Source: three-view drawing plus pictorial views. Frame: mm from the lowest corner of the part. Round coordinates to 2 decimals unless told otherwise and drop trailing zeros. Write each loop counter-clockwise with the first axis right and the second up, starting at its lowest first coordinate (ties: lowest second). Pieces come first, ordered by that corner, then holes. Notation, with made-up numbers: M -7,-5 L 16,-5 A20 ccw 16,4 Z; hole C 1.25,-7 d5. An arc over 180 degrees is marked long. Answer as CSV lines item,"result". Start each with the question number.
Q1. Section query B-B on y = 38. Output: boundary loops of the cut face in (x, z).
Q2. Section query A-A on z = 63.2. Output: boundary loops of the cut face in (x, y).
Q3. First-contact query: pin 1 (12 mm diameter, centred on x = 375, z = 13.2, fed in from -Y). Flat tip, straight axial feed; report the tip coordinate or a pass-through.
Q4. Ray query, probe 1 along X at (y, z) = (11, 63); probe 2 along Z at (x, y) = (25, 18); probe 3 along X at (y, z) = (39, 67.5). Return the intervals inside material, ascending.
Q5. Section query C-C on x = 70. Output: boundary loops of the cut face in (y, z), and give its area (3 significant figures).
Q6. Section query D-D on z = 31. Output: boundary loops of the cut face in (x, y).
Q7. Mould query, pull axis Y, two halves, no side actions, for the marked faces 1, 2, 3 and 4. Classes: pulls with the +Y half, pulls with the -Y half, needs draft (parallel to the pull), parting line crosses it, or undercut.
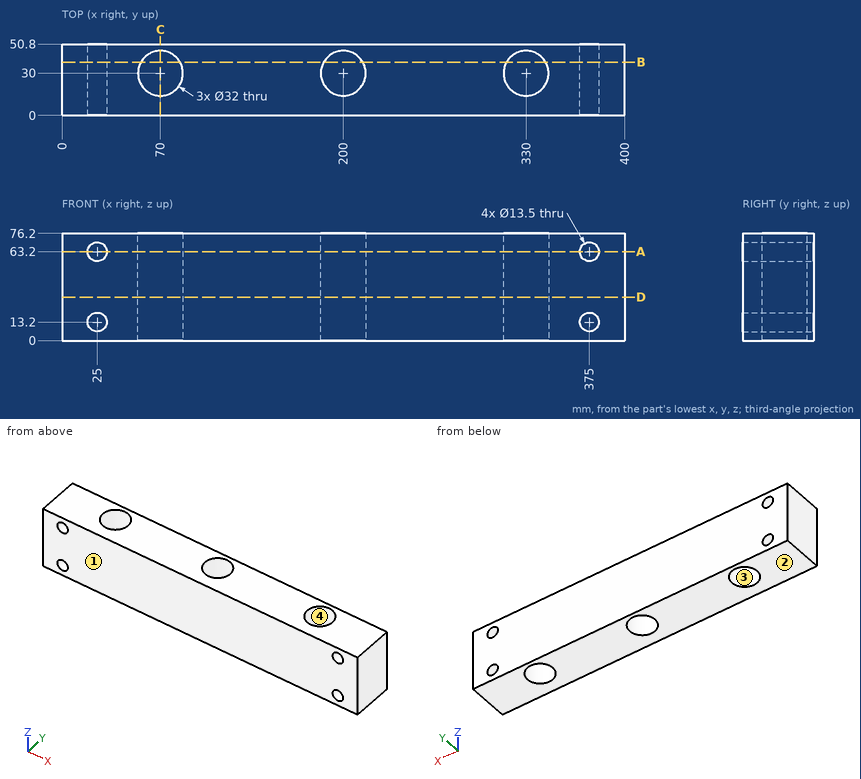
Entries:
1,outline,"M 0,0 L 56.14,0 L 56.14,76.2 L 0,76.2 Z; M 83.86,0 L 186.14,0 L 186.14,76.2 L 83.86,76.2 Z; M 213.86,0 L 316.14,0 L 316.14,76.2 L 213.86,76.2 Z; M 343.86,0 L 400,0 L 400,76.2 L 343.86,76.2 Z; hole C 25,13.2 d13.5; hole C 25,63.2 d13.5; hole C 375,13.2 d13.5; hole C 375,63.2 d13.5"
2,outline,"M 0,0 L 18.25,0 L 18.25,50.8 L 0,50.8 Z; M 31.75,0 L 368.25,0 L 368.25,50.8 L 31.75,50.8 Z; M 381.75,0 L 400,0 L 400,50.8 L 381.75,50.8 Z; hole C 70,30 d32; hole C 200,30 d32; hole C 330,30 d32"
3,pin 1,"passes through"
4,probe 1,"x = 0 to 18.25, 31.75 to 368.25, 381.75 to 400"
4,probe 2,"z = 0 to 6.45, 19.95 to 56.45, 69.95 to 76.2"
4,probe 3,"x = 0 to 19.8, 30.2 to 56.77, 83.23 to 186.77, 213.23 to 316.77, 343.23 to 369.8, 380.2 to 400"
5,outline,"M 0,0 L 14,0 L 14,76.2 L 0,76.2 Z; M 46,0 L 50.8,0 L 50.8,76.2 L 46,76.2 Z"
5,area,"1,430 mm^2"
6,outline,"M 0,0 L 400,0 L 400,50.8 L 0,50.8 Z; hole C 70,30 d32; hole C 200,30 d32; hole C 330,30 d32"
7,face 1,"pulls with the -Y half"
7,face 2,"needs draft"
7,face 3,"undercut"
7,face 4,"undercut"
